Geometry check sheet. Reference: the model listing, model coordinates, mm. Face numbers are marked on the shaded views. A direction names the side the tool comes from. Round coordinates to 2 decimals unless told otherwise and drop trailing zeros. Order: outer loops, then holes, each group sorted by start corner. A loop starts at its lowest first (then second) coordinate and runs counter-clockwise, first axis right, second up. Notation, with made-up numbers: (-7, 52.25) - (36, 52.25) arc R23 cw to (36, 72.25) - close; hole circle Ø7 at (30.25, 52). An arc over 180 degrees is marked (long way). Use a Markdown table: item, result. Add a question column.
(1) Section check C-C on y = -5. Record the boundary of the cut face in (x, z).
(2) Section check A-A on x = 3. Record the boundary of the cut face in (y, z), then the cut area to 3 significant figures.
(3) Section check B-B on y = -15. Give the number of separate pieces and of enclosed holes in the cut face, then the cut area to 3 significant figures.
(4) Section check D-D on x = -21. Record the boundary of the cut face in (y, z).
(5) Gauge pin test, flat ends, axial feed: P1, Ø7.5, axis at x = -7.5, z = 61.5, coming from the +Y side; P2, Ø5, axis at y = -15, z = 27.5, coming from the +X side; P3, Ø5.5, axis at x = 10.4, z = 62, coming from the -Y side; P4, Ø3, axis at y = 15, z = 27.5, coming from the -X side. Record the tip position at first contact, or that the pin passes through.
(6) Thickness scan on line 1 along Y through (x, z) = (-15, 62); line 2 along Z through (x, y) = (9.5, -16); line 3 along Z through (x, y) = (-20, 10). Record the ranges inside material, lowest first. Write a range as [from, to].
(7) Access from +Z, -Z, +X, -X, +Y, -Y to the whole of each face (thin tool, end or side, straight path). Record for the marked faces 1, 2, 3 and 4.
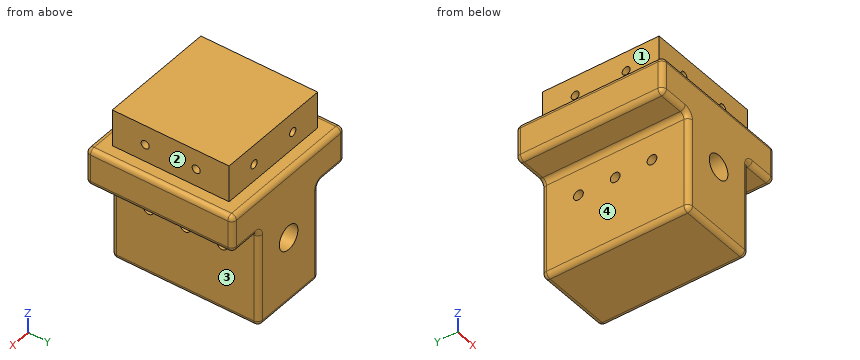
```python
from build123d import *

# Parameters (mm, degrees)
SKETCH2_W                  = 60
SKETCH2_H                  = 60
BOSS_EXTRUDE1_DEPTH        = 70
SKETCH3_OUTSIDE_W          = 84
SKETCH3_OUTSIDE_H          = 84
SKETCH3_OUTSIDE_W_2        = 47.6
SKETCH3_OUTSIDE_H_2        = 47.6
CUT_EXTRUDE1_DEPTH         = 15
M4_TAPPED_HOLE1_AT_2_COUNT = 2
M4_TAPPED_HOLE1_AT_2_PITCH = 20.8
CIRPATTERN1_COUNT          = 4
SKETCH19_R                 = 5
CUT_EXTRUDE2_DEPTH         = 97.953597148
SKETCH21_W                 = 14
SKETCH21_H                 = 60
CUT_EXTRUDE3_DEPTH         = 40
F_4_0MM_DOWEL_HOLE1_D      = 4
FILLET1_R                  = 2


with BuildPart() as part:
    # Sketch2 → Boss-Extrude1 (new body)
    with BuildSketch(Plane.XY):
        Rectangle(SKETCH2_W, SKETCH2_H)
    extrude(amount=BOSS_EXTRUDE1_DEPTH)

    # Sketch3 outside → Cut-Extrude1 (cut)
    with BuildSketch(Plane.XY.offset(70)):
        Rectangle(SKETCH3_OUTSIDE_W, SKETCH3_OUTSIDE_H)
        Rectangle(SKETCH3_OUTSIDE_W_2, SKETCH3_OUTSIDE_H_2, mode=Mode.SUBTRACT)
    extrude(amount=-CUT_EXTRUDE1_DEPTH, mode=Mode.SUBTRACT)

    # Sketch16 → M4 Tapped Hole1 (revolve, cut)
    with BuildSketch(Plane(origin=(23.8, -10.4, 62), x_dir=(0, 0, -1), z_dir=(0, 1, 0))):
        Polygon((0, 0), (0, 12.491420021), (1.65, 11.5), (1.65, 0), align=None)
    m4_tapped_hole1 = revolve(axis=Axis((30.15, -10.4, 62), (-1, 0, 0)), mode=Mode.SUBTRACT)

    # M4 Tapped Hole1 at 2: M4 Tapped Hole1 ×2
    with Locations(*[(0, i * M4_TAPPED_HOLE1_AT_2_PITCH, 0) for i in range(1, M4_TAPPED_HOLE1_AT_2_COUNT)]):
        add(m4_tapped_hole1, mode=Mode.SUBTRACT)

    # CirPattern1: M4 Tapped Hole1 ×4 about axis
    cirpattern1_axis = Axis((0, 0, 70), (0, 0, -1))
    for i in range(1, CIRPATTERN1_COUNT):
        add(m4_tapped_hole1.rotate(cirpattern1_axis, i * 360 / CIRPATTERN1_COUNT), mode=Mode.SUBTRACT)

    # CirPattern1 copy 1 sketch → CirPattern1 copy 1 (revolve, cut)
    with BuildSketch(Plane(origin=(10.4, -23.8, 62), x_dir=(0, 0, -1), z_dir=(1, 0, 0))):
        Polygon((0, 0), (0, 12.491420021), (1.65, 11.5), (1.65, 0), align=None)
    revolve(axis=Axis((10.4, -30.15, 62), (0, 1, 0)), mode=Mode.SUBTRACT)

    # CirPattern1 copy 2 sketch → CirPattern1 copy 2 (revolve, cut)
    with BuildSketch(Plane(origin=(-23.8, -10.4, 62), x_dir=(0, 0, -1), z_dir=(0, -1, 0))):
        Polygon((0, 0), (0, 12.491420021), (1.65, 11.5), (1.65, 0), align=None)
    revolve(axis=Axis((-30.15, -10.4, 62), (1, 0, 0)), mode=Mode.SUBTRACT)

    # CirPattern1 copy 3 sketch → CirPattern1 copy 3 (revolve, cut)
    with BuildSketch(Plane(origin=(-10.4, 23.8, 62), x_dir=(0, 0, -1), z_dir=(-1, 0, 0))):
        Polygon((0, 0), (0, 12.491420021), (1.65, 11.5), (1.65, 0), align=None)
    revolve(axis=Axis((-10.4, 30.15, 62), (0, -1, 0)), mode=Mode.SUBTRACT)

    # Sketch19 → Cut-Extrude2 (cut, through all)
    with BuildSketch(Plane(origin=(0, 30, 0), x_dir=(1, 0, 0), z_dir=(0, 1, 0))):
        with Locations(Location((0, -27.5, 0), (0, 0, 270))):
            Circle(SKETCH19_R)
    extrude(amount=-CUT_EXTRUDE2_DEPTH, mode=Mode.SUBTRACT)

    # Sketch21 → Cut-Extrude3 (cut)
    with BuildSketch(Plane(origin=(0, 0, 0), x_dir=(-1, 0, 0), z_dir=(0, 0, -1))):
        with Locations((-23, 0)):
            Rectangle(SKETCH21_W, SKETCH21_H)
    cut_extrude3 = extrude(amount=-CUT_EXTRUDE3_DEPTH, mode=Mode.SUBTRACT)

    # Mirror1: Cut-Extrude3 across plane
    add(cut_extrude3.mirror(Plane(origin=(0, 0, 0), x_dir=(0, 0, 1), z_dir=(1, 0, 0))), mode=Mode.SUBTRACT)

    # Ø4.0mm Dowel Hole1 (through all)
    with Locations(Plane.ZY.offset(16)):
        with Locations((27.5, 15), (27.5, 0), (27.5, -15)):
            Hole(F_4_0MM_DOWEL_HOLE1_D / 2)

    # Fillet1
    fillet1_edges = [part.edges().sort_by_distance(p)[0] for p in [
        (0, -30, 0),
        (-16, 0, 0),
        (-16, -30, 20),
        (-16, 30, 20),
        (-30, 0, 40),
        (-23, -30, 40),
        (-16, 0, 40),
        (-23, 30, 40),
        (30, -30, 47.5),
        (-30, -30, 47.5),
        (0, -30, 55),
        (-30, 30, 47.5),
        (30, 30, 47.5),
        (30, 0, 55),
        (0, 30, 55),
        (-30, 0, 55),
        (0, 30, 0),
        (30, 0, 40),
        (23, 30, 40),
        (16, 0, 40),
        (16, 30, 20),
        (23, -30, 40),
        (16, -30, 20),
        (16, 0, 0),
    ]]
    fillet(fillet1_edges, radius=FILLET1_R)


solid = part.part
```
Check sheet entries:
| question | item | result |
|---|---|---|
| 1 | outline | (-30, 42) arc R2 ccw to (-28, 40) - (-18, 40) arc R2 cw to (-16, 38) - (-16, 2) arc R2 ccw to (-14, 0) - (14, 0) arc R2 ccw to (16, 2) - (16, 38) arc R2 cw to (18, 40) - (28, 40) arc R2 ccw to (30, 42) - (30, 53) arc R2 ccw to (28, 55) - (23.8, 55) - (23.8, 70) - (-23.8, 70) - (-23.8, 55) - (-28, 55) arc R2 ccw to (-30, 53) - close; hole circle Ø10 at (0, 27.5) |
| 2 | outline | (-30, 2) arc R2 ccw to (-28, 0) - (28, 0) arc R2 ccw to (30, 2) - (30, 23.5) - (-30, 23.5) - close; (-30, 31.5) - (30, 31.5) - (30, 53) arc R2 ccw to (28, 55) - (23.8, 55) - (23.8, 70) - (-23.8, 70) - (-23.8, 55) - (-28, 55) arc R2 ccw to (-30, 53) - close |
| 2 | area | 3,530 mm2 |
| 3 | separate pieces | 2 |
| 3 | enclosed holes | 2 |
| 3 | area | 2,710 mm2 |
| 4 | outline | (-30, 42) arc R2 ccw to (-28, 40) - (28, 40) arc R2 ccw to (30, 42) - (30, 53) arc R2 ccw to (28, 55) - (23.8, 55) - (23.8, 70) - (-23.8, 70) - (-23.8, 55) - (-28, 55) arc R2 ccw to (-30, 53) - close; hole circle Ø3.3 at (-10.4, 62); hole circle Ø3.3 at (10.4, 62) |
| 5 | P1 | stops at y = 23.8 |
| 5 | P2 | stops at x = 16 |
| 5 | P3 | stops at y = -23.8 |
| 5 | P4 | passes through |
| 6 | line 1 | y = [-23.8, -12.05], [-8.75, 8.75], [12.05, 23.8] |
| 6 | line 2 | z = [0, 25.77], [29.23, 60.62], [63.38, 70] |
| 6 | line 3 | z = [40, 60.4], [63.6, 70] |
| 7 | face 1 | +Z, -X, +Y, -Y |
| 7 | face 2 | +Z, +X, +Y, -Y |
| 7 | face 3 | -Z, +X, +Y, -Y |
| 7 | face 4 | -Z, -X, +Y, -Y |
